```python
from build123d import *

# Parameters (mm, degrees)
BOSS_EXTRUDE1_DEPTH  = 3.175
FILLET1_R            = 12.7
SKETCH2_W            = 3.175
SKETCH2_H            = 1.5875
CABLE_TIE_HOLE_DEPTH = 160.383735055


with BuildPart() as part:
    # Sketch1 → Boss-Extrude1 (new, symmetric)
    with BuildSketch(Plane(origin=(0, 0, 0), x_dir=(0, 0, -1), z_dir=(1, 0, 0))):
        Polygon((12.7, -69.53755182), (12.7, -158.75), (6.35, -158.75), (6.35, -152.4), (-12.7, -152.4), (-12.7, 12.7), (12.7, 12.7), align=None)
    extrude(amount=BOSS_EXTRUDE1_DEPTH, both=True)

    # Fillet1
    fillet1_edges = [part.edges().sort_by_distance(p)[0] for p in [
        (0, 12.7, -12.7),
        (0, 12.7, 12.7),
    ]]
    fillet(fillet1_edges, radius=FILLET1_R - 0.0001)  # a hair under: the kernel refuses the full size

    # Sketch2 → Cable-tie hole (cut, through all)
    with BuildSketch(Plane(origin=(3.175, 0, 0), x_dir=(0, 0, -1), z_dir=(1, 0, 0))):
        with Locations((-3.175, -145.25625)):
            Rectangle(SKETCH2_W, SKETCH2_H)
    extrude(amount=-CABLE_TIE_HOLE_DEPTH, mode=Mode.SUBTRACT)


solid = part.part
```
Source: CAD feature listing. Evaluate the final solid. Frame: model axes, mm. A direction names the side the tool comes from. Coordinates: 2 decimals unless noted, no trailing zeros. Loops run counter-clockwise (first coordinate to the right, second up) from the corner with the lowest first, then second, coordinate; pieces in that order, holes last. Notation, with made-up numbers: (-19.75, 12) -> (-10.75, 12) arc R18 ccw to (-10.75, 42) -> close; hole circle Ø5 at (-15.75, 57.25). An arc over 180 degrees is marked (long way). One line per item, written item: value. Start each with the question number.
Q1. Line query: line 1 along Z through (x, y) = (2.75, -146); line 2 along Y through (x, z) = (-2, 3.5); line 3 along Y through (x, z) = (-1, 7.75). Output: solid intervals per line, ascending.
Q2. Contact query for flat-ended pins moving along their axis: P1, Ø1.6, axis at x = 0, z = 3, coming from the -Y side; P2, Ø1, axis at x = 1, z = 2.5, coming from the +Y side; P3, Ø1, axis at x = 2, z = 8.5, coming from the +Y side. Output: stop coordinate, or through.
Q3. Section query B-B, the plane z = 8.5. Return the cut outline in (x, y) (3 decimals), and give its area (3 significant figures).
Q4. Set-up query: faces 4 (the face through (0, -146.05, 3)), 5 (the face through (0.04, 8.88, -9.08)), 6 (the face through (0, -152.4, 3)). Return all of +Z, -Z, +X, -X, +Y, -Y with unobstructed straight access to the full face (end or side cutting, diameter ignored); none if empty.
Q5. Mould query, pull axis Z, two halves, no side actions, for faces 1 (the face through (0, -156, -6.35)), 2 (the face through (-3.175, -72, 0)), 3 (the face through (0, -144.462, 3)). Classes: pulls with the +Z half, pulls with the -Z half, needs draft (parallel to the pull), parting line crosses it, or undercut.
Q6. Section query C-C, the plane z = -2. Return the cut outline in (x, y) (3 decimals).
Results:
1. line 1: -12.7 to 1.59, 4.76 to 12.7
1. line 2: -152.4 to -146.05, -144.46 to 12.21
1. line 3: -152.4 to 10.06
2. P1: y = -152.4
2. P2: y = 12.54
2. P3: y = 9.86
3. outline: (-3.175, -152.4) -> (3.175, -152.4) -> (3.175, 9.436) -> (-3.175, 9.436) -> close
3. area: 1,030 mm^2
4. face 4: +X, -X
4. face 5: -Z, +X, -X, +Y
4. face 6: +Z, +X, -X, -Y
5. face 1: pulls with the +Z half
5. face 2: needs draft
5. face 3: undercut
6. outline: (-3.175, -152.4) -> (3.175, -152.4) -> (3.175, 12.542) -> (-3.175, 12.542) -> close
